Verification items for the finished model (mm, model axes). Face numbers are marked on the shaded views. A direction names the side the tool comes from. Give positions to 0.01 mm unless a question says otherwise; leave off trailing zeros. Order: outer loops, then holes, each group sorted by start corner. A loop starts at its lowest first (then second) coordinate and runs counter-clockwise, first axis right, second up.
from build123d import *

# Parameters (mm, degrees)
BASEPLATE_SKETCH_R   = 2.65
BASEPLATE_SKETCH_R_2 = 6.25
BOSS_EXTRUDE1_DEPTH  = 6.35
SKETCH3_R            = 1.6
CUT_EXTRUDE2_DEPTH   = 6.35


with BuildPart() as part:
    # Baseplate Sketch → Boss-Extrude1 (new body)
    with BuildSketch(Plane(origin=(0, 0, 0), x_dir=(1, 0, 0), z_dir=(0, 1, 0))):
        with BuildLine():
            ThreePointArc((17.5, 30.310889132), (0, 35), (-17.5, 30.310889132))
            Line((-17.5, 30.310889132), (-15, 25.980762114))
            ThreePointArc((-15, 25.980762114), (-25.980762114, 15), (-30, 0))
            Line((-30, 0), (-35, 0))
            ThreePointArc((-35, 0), (-30.310889132, -17.5), (-17.5, -30.310889132))
            Line((-17.5, -30.310889132), (-15, -25.980762114))
            ThreePointArc((-15, -25.980762114), (0, -30), (15, -25.980762114))
            Line((15, -25.980762114), (17.5, -30.310889132))
            ThreePointArc((17.5, -30.310889132), (30.310889132, -17.5), (35, 0))
            Line((35, 0), (30, 0))
            ThreePointArc((30, 0), (25.980762114, 15), (15, 25.980762114))
            Line((15, 25.980762114), (17.5, 30.310889132))
        make_face()
        with Locations(Location((0, 25, 0), (0, 0, 270))):
            Circle(BASEPLATE_SKETCH_R, mode=Mode.SUBTRACT)
        with Locations(Location((-21.650635095, -12.5, 0), (0, 0, 270))):
            Circle(BASEPLATE_SKETCH_R, mode=Mode.SUBTRACT)
        with Locations(Location((0, 0, 0), (0, 0, 270))):
            Circle(BASEPLATE_SKETCH_R_2, mode=Mode.SUBTRACT)
        with Locations(Location((21.650635095, -12.5, 0), (0, 0, 270))):
            Circle(BASEPLATE_SKETCH_R, mode=Mode.SUBTRACT)
    extrude(amount=BOSS_EXTRUDE1_DEPTH)

    # Sketch3 → Cut-Extrude2 (cut)
    with BuildSketch(Plane(origin=(0, 6.35, 0), x_dir=(1, 0, 0), z_dir=(0, 1, 0))):
        with Locations(Location((-8.127648415, -4.6925, 0), (0, 0, 270))):
            Circle(SKETCH3_R)
        with Locations(Location((0, -9.385, 0), (0, 0, 270))):
            Circle(SKETCH3_R)
        with Locations(Location((-8.127648415, 4.6925, 0), (0, 0, 270))):
            Circle(SKETCH3_R)
        with Locations(Location((0, 9.385, 0), (0, 0, 270))):
            Circle(SKETCH3_R)
        with Locations(Location((8.127648415, 4.6925, 0), (0, 0, 270))):
            Circle(SKETCH3_R)
        with Locations(Location((8.127648415, -4.6925, 0), (0, 0, 270))):
            Circle(SKETCH3_R)
    extrude(amount=-CUT_EXTRUDE2_DEPTH, mode=Mode.SUBTRACT)


solid = part.part
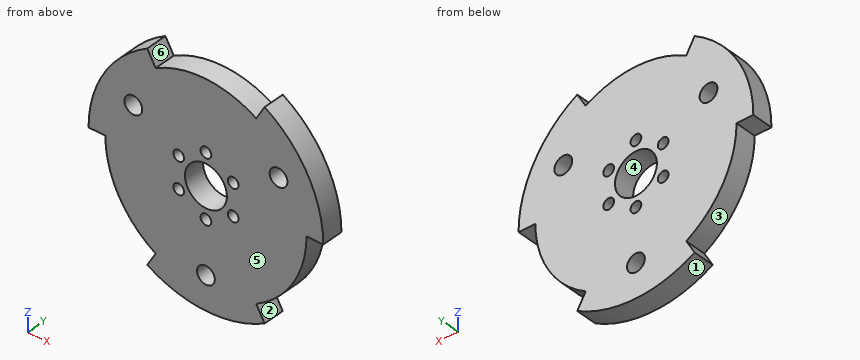
(1) Section check D-D, the plane z = -9. Enter the section's corners in (x, y).
Solved:
outline: (-28.62, 0) - (-1.55, 0) - (-1.55, 6.35) - (-28.62, 6.35) - close; (1.55, 0) - (28.62, 0) - (28.62, 6.35) - (1.55, 6.35) - close
(2) Go/stop test with flat-tipped pins: pin 1 (1.5 mm diameter, centred on y = 1.5, z = 23.5, fed in from +X); pin 2 (3 mm diameter, centred on y = 2.5, z = 15.5, fed in from -X); pin 3 (4 mm diameter, centred on x = 0, z = -9.385, fed in from +Y); pin 4 (2 mm diameter, centred on x = -6.5, y = 4.5, fed in from -Z). Record where each tip stops, or that it passes through.
Solved:
pin 1: stops at x = 26.6
pin 2: stops at x = -32.08
pin 3: stops at y = 6.35
pin 4: stops at z = -34.57
(3) Section check A-A, the plane x = 0. Enter the section's corners in (y, z) (3 decimals), then the cut area to 3 significant figures.
Solved:
outline: (0, -35) - (6.35, -35) - (6.35, -27.65) - (0, -27.65) - close; (0, -22.35) - (6.35, -22.35) - (6.35, -10.985) - (0, -10.985) - close; (0, -7.785) - (6.35, -7.785) - (6.35, -6.25) - (0, -6.25) - close; (0, 6.25) - (6.35, 6.25) - (6.35, 7.785) - (0, 7.785) - close; (0, 10.985) - (6.35, 10.985) - (6.35, 30) - (0, 30) - close
area: 259 mm2
(4) Set-up check for the marked faces 5 and 6: record each of +Z, -Z, +X, -X, +Y, -Y from which the full face is reachable in a straight line by a thin tool's end or side.
Solved:
face 5: +Z, -Z, +X, -X, -Y
face 6: +Z, +Y, -Y
(5) Section check B-B, the plane z = 2. Enter the section's corners in (x, y).
Solved:
outline: (-34.94, 0) - (-5.92, 0) - (-5.92, 6.35) - (-34.94, 6.35) - close; (5.92, 0) - (34.94, 0) - (34.94, 6.35) - (5.92, 6.35) - close
(6) Scan lines: line 1 (Z direction, x = -0.5, y = 3.75); line 2 (X direction, y = 5.25, z = -5.5); line 3 (X direction, y = 3.5, z = 11.5). Record each from-to range of solid material in increasing order.
Solved:
line 1: z = -35 to -27.6, -22.4 to -10.9, -7.87 to -6.23, 6.23 to 7.87, 10.9 to 30
line 2: x = -29.49 to -9.51, -6.75 to -2.97, 2.97 to 6.75, 9.51 to 29.49
line 3: x = -33.06 to -24.1, -19.2 to 19.2, 24.1 to 33.06
(7) Release check for a two-part mould opening along X. For the marked faces 1, 2, 3 and 4 record: pulls with the +X half, pulls with the -X half, needs draft (parallel to the pull), parting line crosses it, or undercut.
Solved:
face 1: parting line crosses it
face 2: pulls with the +X half
face 3: pulls with the -X half
face 4: undercut
(8) Section check C-C, the plane y = 1.5. Give the number of separate pieces and of enclosed holes in the cut face, then the cut area to 3 significant figures.
Solved:
separate pieces: 1
enclosed holes: 10
area: 3,100 mm2
